Check sheet for the modelled part. Datum: model origin and axes. Units: mm. Round coordinates to 2 decimals unless told otherwise and drop trailing zeros. Order: outer loops, then holes, each group sorted by start corner. A loop starts at its lowest first (then second) coordinate and runs counter-clockwise, first axis right, second up. Notation, with made-up numbers: (43.5, 8.5) -> (79.5, 8.5) arc R22 ccw to (79.5, 24.5) -> close; hole circle Ø3 at (-37, 43). An arc over 180 degrees is marked (long way). Use CSV: the item, a comma, the result in double quotes.
```python
from build123d import *

# Parameters (mm, degrees)
F0_W      = 82.55
F0_H      = 38.1
F0_R      = 9.8
F0_R_2    = 11
F1_DEPTH  = 12.954
F1_FACE_W = 82.55
F1_FACE_H = 12.954
F2_DEPTH  = 0.254


with BuildPart() as f1:
    # F0 (on Top) → F1 (new body)
    with BuildSketch(Plane.XY):
        with Locations((41.275, 19.05)):
            Rectangle(F0_W, F0_H)
        with Locations((12.531688, 19.761506)):
            Circle(F0_R, mode=Mode.SUBTRACT)
        with Locations((41.932955, 19.279519)):
            Circle(F0_R_2, mode=Mode.SUBTRACT)
        with Locations((71.816206, 19.279519)):
            Circle(F0_R, mode=Mode.SUBTRACT)
    extrude(amount=F1_DEPTH)

    # F1_face (on face) → F2 (cut)
    with BuildSketch(Plane(origin=(41.275, 0, 6.477), x_dir=(1, 0, 0), z_dir=(0, -1, 0))):
        Rectangle(F1_FACE_W, F1_FACE_H)
    extrude(amount=-F2_DEPTH, mode=Mode.SUBTRACT)


solid = f1.part
```
Q1. Sectioned sample at D-D, the plane x = 21. Enter the section's corners in (y, z), then the cut area to 3 significant figures.
Result sheet:
outline,"(0.25, 0) -> (14.83, 0) -> (14.83, 12.95) -> (0.25, 12.95) -> close; (24.69, 0) -> (38.1, 0) -> (38.1, 12.95) -> (24.69, 12.95) -> close"
area,"362 mm^2"
Q2. Mould release check, pull along X, two halves, no side actions. Record for faces 1 (the face through (0, 19, 6)), 2 (the face through (80.87, 15.53, 6.39)), 3 (the face through (41, 38.1, 6)): pulls with the +X half, pulls with the -X half, needs draft (parallel to the pull), parting line crosses it, or undercut.
Result sheet:
face 1,"pulls with the -X half"
face 2,"undercut"
face 3,"needs draft"
Q3. Sectioned sample at A-A, the plane x = 34. Enter the section's corners in (y, z).
Result sheet:
outline,"(0.25, 0) -> (11.66, 0) -> (11.66, 12.95) -> (0.25, 12.95) -> close; (26.9, 0) -> (38.1, 0) -> (38.1, 12.95) -> (26.9, 12.95) -> close"
Q4. Scan lines: L1, parallel to X at y = 19.5, z = 6; L2, parallel to X at y = 14, z = 6; L3, parallel to Y at x = 72, z = 1.25. Record each from-to range of solid material in increasing order.
Result sheet:
L1,"x = 0 to 2.74, 22.33 to 30.94, 52.93 to 62.02, 81.61 to 82.55"
L2,"x = 0 to 4.6, 20.46 to 32.28, 51.58 to 63.56, 80.07 to 82.55"
L3,"y = 0.25 to 9.48, 29.08 to 38.1"
Q5. Sectioned sample at B-B, the plane y = 11.5. Enter the section's corners in (x, z), then the cut area to 3 significant figures.
Result sheet:
outline,"(0, 0) -> (7.26, 0) -> (7.26, 12.95) -> (0, 12.95) -> close; (17.8, 0) -> (34.16, 0) -> (34.16, 12.95) -> (17.8, 12.95) -> close; (49.71, 0) -> (65.86, 0) -> (65.86, 12.95) -> (49.71, 12.95) -> close; (77.78, 0) -> (82.55, 0) -> (82.55, 12.95) -> (77.78, 12.95) -> close"
area,"577 mm^2"
Q6. Sectioned sample at C-C, the plane z = 6.5. Enter the section's corners in (x, y), then the cut area to 3 significant figures.
Result sheet:
outline,"(0, 0.25) -> (82.55, 0.25) -> (82.55, 38.1) -> (0, 38.1) -> close; hole circle Ø19.6 at (12.53, 19.76); hole circle Ø22 at (41.93, 19.28); hole circle Ø19.6 at (71.82, 19.28)"
area,"2,140 mm^2"
